Job drawing, mm, ordinate dimensions from the low corner. One solid piece. A direction names the side the tool comes from. Coordinates: 2 decimals unless noted, no trailing zeros. Loops run counter-clockwise (first coordinate to the right, second up) from the corner with the lowest first, then second, coordinate; pieces in that order, holes last. Notation, with made-up numbers: (81, -39.75) -> (134, -39.75) arc R12 ccw to (134, -27.75) -> close; hole circle Ø2 at (30, 49.25). An arc over 180 degrees is marked (long way). Answer as CSV lines item,"result". Start each with the question number.
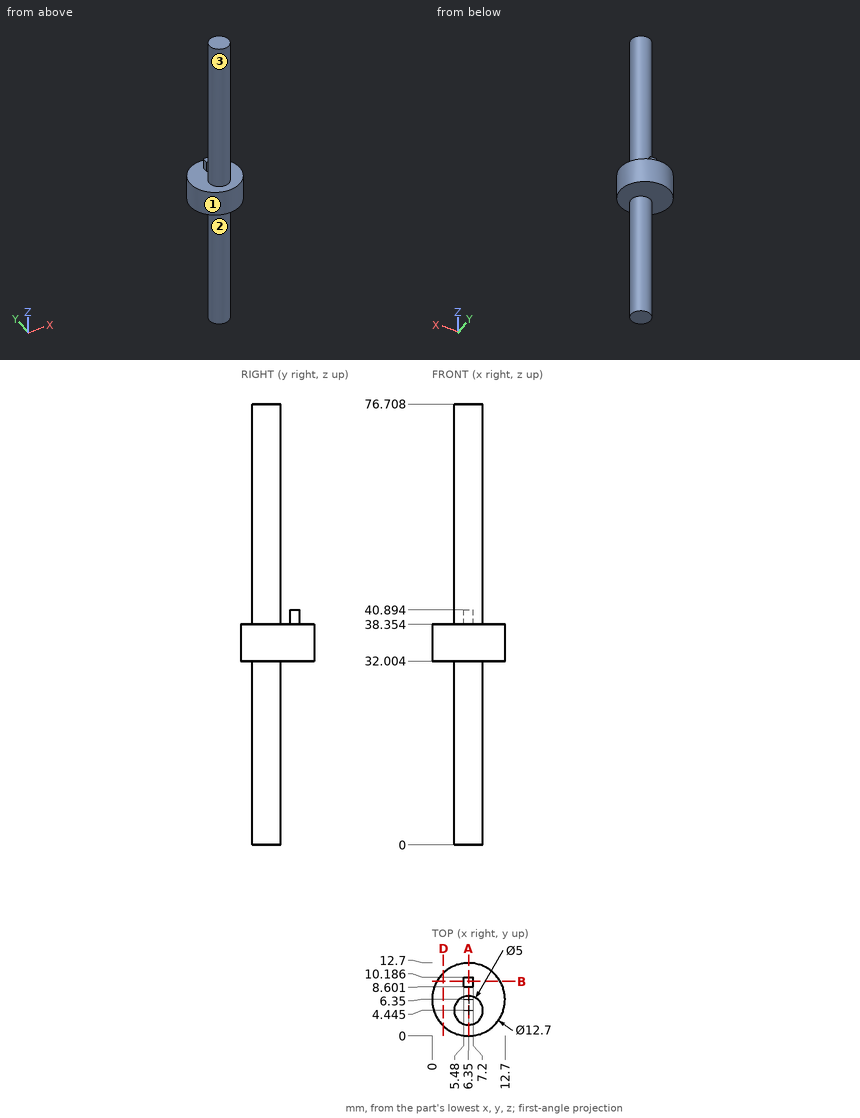
Q1. Probe probe 1 along Z at (x, y) = (3, 5.75); probe 2 along Z at (x, y) = (7, 10); probe 3 along X at (y, z) = (6, 35.5). List the from-to ranges inside material, lowest first. Write a range as from..to.
Q2. Saw through at B-B (y = 9.5). List the corners of the cut face in (x, z).
Q3. Saw through at A-A (x = 6.35). List the corners of the cut face in (y, z) (1 decimal).
Q4. Saw through at D-D (x = 2). List the corners of the cut face in (y, z).
Q5. Which spindle directions (+Z, -Z, +X, -X, +Y, -Y) get a long thin tool onto all of the face, cutting with end or side? Do the marked faces 1, 2 and 3. Say none if no direction does.
Q6. Pin check, flat tips, straight feed: pin 1 Ø4 at (y, z) = (3.5, 29) entering from -X; pin 2 Ø1.3 at (x, y) = (6, 9.5) entering from +Z; pin 3 Ø2 at (y, z) = (2.5, 22) entering from -X (1 decimal). Stop position of each tip, or through.
Ans:
1,probe 1,"z = 32..38.35"
1,probe 2,"z = 32..40.89"
1,probe 3,"x = 0.01..12.69"
2,outline,"(0.84, 32) -> (11.86, 32) -> (11.86, 38.35) -> (7.2, 38.35) -> (7.2, 40.89) -> (5.48, 40.89) -> (5.48, 38.35) -> (0.84, 38.35) -> close"
3,outline,"(0, 32) -> (1.9, 32) -> (1.9, 0) -> (6.9, 0) -> (6.9, 32) -> (12.7, 32) -> (12.7, 38.4) -> (10.2, 38.4) -> (10.2, 40.9) -> (8.6, 40.9) -> (8.6, 38.4) -> (6.9, 38.4) -> (6.9, 76.7) -> (1.9, 76.7) -> (1.9, 38.4) -> (0, 38.4) -> close"
4,outline,"(1.72, 32) -> (10.98, 32) -> (10.98, 38.35) -> (1.72, 38.35) -> close"
5,face 1,"+Z, -Z"
5,face 2,"-Z"
5,face 3,"+Z"
6,pin 1,"stops at x = 3.85"
6,pin 2,"stops at z = 40.89"
6,pin 3,"stops at x = 4"
